Here's how the part is built. I have some questions about the finished solid (model axes, mm). A direction names the side the tool comes from. Coordinates: 2 decimals unless noted, no trailing zeros. Loops run counter-clockwise (first coordinate to the right, second up) from the corner with the lowest first, then second, coordinate; pieces in that order, holes last. Notation, with made-up numbers: M 11,67.25 L 25,67.25 A28 ccw 25,96.25 Z; hole C 49,7 d7. An arc over 180 degrees is marked long. Use one line per item in the form item = value. Start each with the question number.
(1) Please list where these lines run through material, in increasing order: L1, parallel to X at y = -1, z = 0.5; L2, parallel to Y at x = -4, z = 1.1; L3, parallel to X at y = -0.25, z = 1.6.
(2) Thinking about a two-plate mould opening in Y: for faces 1 (the cylindrical face through (10.05, 0.65, 4.12)), 2 (the flat face through (-11.938, 0, 2)), 3 (the flat face through (10.541, 0, 1)), 4 (the cylindrical face through (-2.694, 0.067, 0.901)), which applies, +Y half, -Y half, draft (parallel to the pull), parting line (faces both ways), or undercut?
(3) Imagine slicing it at A-A, the plane z = 1.25. Please give me the cut outline in (x, y), and give its area (3 significant figures).
(4) On a 3-axis mill with a long thin cutter (end or side, diameter ignored), from which of +Z, -Z, +X, -X, +Y, -Y can I reach the whole of each face in a straight line? I mean faces 5 (the flat face through (-8, 0, 5.004)), 6 (the cylindrical face through (-10.05, -0.72, 4.12)), 7 (the flat face through (0, 2.54, 1)). Say none if no direction works.
(5) Imagine slicing it at B-B, the plane y = 0.5. Please give me the cut outline in (x, z).
(6) Imagine slicing it at D-D, the plane z = 4.05. Please give me the cut outline in (x, y), and give its area (3 significant figures).
(7) Will this pin go through, and if not, where does the flat tip stop? P1, Ø1.5, axis at x = 4.5, y = -2.5, coming from the +Z side.
(8) Imagine slicing it at C-C, the plane x = 4. Please give me the cut outline in (y, z), and give its area (3 significant figures).
```python
from build123d import *

# Parameters (mm, degrees)
F0_W     = 23.876
F0_H     = 7.874
F1_DEPTH = 3.2512
F2_W     = 21.082
F2_H     = 5.08
F3_DEPTH = 1.778
F4_R     = 2.413
F5_DEPTH = 1.7526
F6_R     = 1.524
F7_DEPTH = 1.778


with BuildPart() as f1:
    # F0 (on Top) → F1 (new body)
    with BuildSketch(Plane.XY):
        Rectangle(F0_W, F0_H)
    extrude(amount=F1_DEPTH)

    # F2 (on face) → F3 (cut)
    with BuildSketch(Plane(origin=(0, 0, 0), x_dir=(1, 0, 0), z_dir=(0, 0, -1))):
        Rectangle(F2_W, F2_H)
    extrude(amount=-F3_DEPTH, mode=Mode.SUBTRACT)

    # F4 (on face) → F5 (join)
    with BuildSketch(Plane.XY.offset(3.2512)):
        with BuildLine():
            ThreePointArc((-5.334, 0), (-7.747, 2.413), (-10.16, 0))
            ThreePointArc((-10.16, 0), (-7.747, -2.413), (-5.334, 0))
        make_face()
        with Locations((-9.4e-05, -0.038094)):
            Circle(F4_R)
        with Locations((7.746813, -0.076188)):
            Circle(F4_R)
    extrude(amount=F5_DEPTH)

    # F6 (on face) → F7 (join)
    with BuildSketch(Plane(origin=(0, 0, 1.778), x_dir=(1, 0, 0), z_dir=(0, 0, -1))):
        with BuildLine():
            ThreePointArc((-2.6924, 0), (-4.2164, 1.524), (-5.7404, 0))
            ThreePointArc((-5.7404, 0), (-4.2164, -1.524), (-2.6924, 0))
        make_face()
        with Locations((4.2164, 0)):
            Circle(F6_R)
    extrude(amount=F7_DEPTH)


solid = f1.part
```
Answer:
q1.L1 = -11.94 to -10.54, -5.37 to -3.07, 3.07 to 5.37, 10.54 to 11.94
q1.L2 = -3.94 to -2.54, -1.51 to 1.51, 2.54 to 3.94
q1.L3 = -11.94 to -10.54, -5.72 to -2.71, 2.71 to 5.72, 10.54 to 11.94
q2.face_1 = parting line
q2.face_2 = draft
q2.face_3 = undercut
q2.face_4 = undercut
q3.outline = M -11.94,-3.94 L 11.94,-3.94 L 11.94,3.94 L -11.94,3.94 Z; C -4.22,0 d3.05; C 4.22,0 d3.05; hole M -10.54,-2.54 L 10.54,-2.54 L 10.54,2.54 L -10.54,2.54 Z
q3.area = 95.5 mm²
q4.face_5 = +Z, +X, -X, +Y, -Y
q4.face_6 = +Z
q4.face_7 = -Z
q5.outline = M -11.94,0 L -10.54,0 L -10.54,1.78 L -5.66,1.78 L -5.66,0 L -2.78,0 L -2.78,1.78 L 2.78,1.78 L 2.78,0 L 5.66,0 L 5.66,1.78 L 10.54,1.78 L 10.54,0 L 11.94,0 L 11.94,3.25 L 10.09,3.25 L 10.09,5 L 5.4,5 L 5.4,3.25 L 2.35,3.25 L 2.35,5 L -2.35,5 L -2.35,3.25 L -5.39,3.25 L -5.39,5 L -10.11,5 L -10.11,3.25 L -11.94,3.25 Z
q6.outline = C -7.75,0 d4.83; C 0,-0.04 d4.83; C 7.75,-0.08 d4.83
q6.area = 54.9 mm²
q7.P1 = 3.25
q8.outline = M -3.94,0 L -2.54,0 L -2.54,1.78 L -1.51,1.78 L -1.51,0 L 1.51,0 L 1.51,1.78 L 2.54,1.78 L 2.54,0 L 3.94,0 L 3.94,3.25 L -3.94,3.25 Z
q8.area = 21.9 mm²
